Autodesk Inventor part; units mm, degrees
ref_plane "YZ Plane" through (0, 0, 0) normal (1, 0, 0) x (0, 1, 0)
ref_plane "XZ Plane" through (0, 0, 0) normal (0, 1, 0) x (-1, 0, 0)
ref_plane "XY Plane" through (0, 0, 0) normal (0, 0, 1) x (1, 0, 0)
sketch "スケッチ1" plane through (0, 0, 0) normal (0, 0, 1) x (1, 0, 0)
  circle A0 centre (0, 0) radius 2.75
  dimension "d0" = 5.5
extrude "押し出し1" add sketch "スケッチ1" along normal blind 3.6
sketch "スケッチ2" plane through (0, 0, 3.6) normal (0, 0, 1) x (1, 0, 0)
  circle A0 centre (0, 0) radius 1.5
  dimension "d3" = 3
extrude "押し出し2" add sketch "スケッチ2" along normal blind 15
thread "ねじ1"
sketch "スケッチ3" plane through (0, 0, 0) normal (0, 0, -1) x (-1, 0, 0)
  line L0 (0, -1.4434) -> (-1.25, -0.7217)
  line L1 (-1.25, -0.7217) -> (-1.25, 0.7217)
  line L2 (-1.25, 0.7217) -> (0, 1.4434)
  line L3 (0, 1.4434) -> (1.25, 0.7217)
  line L4 (1.25, 0.7217) -> (1.25, -0.7217)
  line L5 (1.25, -0.7217) -> (0, -1.4434)
  point P0 (0, 0)
  point P1 (0, 0)
  dimension "d8" = 2.5
extrude "押し出し3" cut sketch "スケッチ3" against normal blind 2
properties part number "Bolt_M3_15_for_SetCollar_d6" material "ステンレス鋼"
The model under review builds one solid part; all positions refer to its coordinate system, in mm. A direction names the side the tool comes from. Coordinates: 2 decimals unless noted, no trailing zeros. Write each loop counter-clockwise with the first axis right and the second up, starting at its lowest first coordinate (ties: lowest second). Pieces come first, ordered by that corner, then holes. Notation, with made-up numbers: (21.5, -17) - (65.5, -17) arc R19 cw to (65.5, 6) - close; hole circle Ø6 at (8.5, -38). An arc over 180 degrees is marked (long way). Answer in a Markdown table with one row per item. Add a question column.
Q1. Consider section B-B on x = 0.75. Give the boundary of the cut face in (y, z), then the cut area to 3 significant figures.
Q2. To check wall thickness, follow line 1 along Z through (x, y) = (-0.85, -1.55); line 2 along Z through (x, y) = (0.25, 0.45); line 3 along X through (y, z) = (0.4, 9.5). State the ranges of each line that lie inside material, in increasing order. Write a range as from..to.
Q3. Clearance check with a flat-ended pin moving along its axis: pin 1 (0.8 mm diameter, centred on x = 0, y = 0.5, fed in from -Z). State where the tip first meets the part, or that it passes through.
Q4. Consider section C-C on z = 8.75. Give the boundary of the cut face in (x, y), then the cut area to 3 significant figures.
Q5. For faces 1 (the face through (1.25, 0, 1)), 2 (the face through (0.6, 1.3, 0)), list the 3-axis set-ups (+Z, -Z, +X, -X, +Y, -Y) from which the entire face can be reached by the end or side of a thin tool; tool diameter is ignored.
Q6. Draft analysis for pull direction X (two halves, no side actions). For faces 3 (the face through (0.616, -1.088, 0.986)), 4 (the face through (-1.5, -0.07, 11)), 5 (the face through (1.2, -1.2, 3.6)), state which applies: +X half, -X half, draft (parallel to the pull), parting line (faces both ways), or undercut.
Q7. Consider section A-A on y = 0. Give the boundary of the cut face in (x, z), then the cut area to 3 significant figures.
Q8. Consider section D-D on x = -1.8. Give the boundary of the cut face in (y, z), then the cut area to 3 significant figures.
Answers below:
| question | item | result |
|---|---|---|
| 1 | outline | (-2.65, 0) - (-1.01, 0) - (-1.01, 2) - (1.01, 2) - (1.01, 0) - (2.65, 0) - (2.65, 3.6) - (1.3, 3.6) - (1.3, 18.6) - (-1.3, 18.6) - (-1.3, 3.6) - (-2.65, 3.6) - close |
| 1 | area | 54.0 mm² |
| 2 | line 1 | 0..3.6 |
| 2 | line 2 | 2..18.6 |
| 2 | line 3 | -1.45..1.45 |
| 3 | pin 1 | z = 2 |
| 4 | outline | circle Ø3 at (0, 0) |
| 4 | area | 7.07 mm² |
| 5 | face 1 | -Z |
| 5 | face 2 | -Z, +X, -X, +Y, -Y |
| 6 | face 3 | undercut |
| 6 | face 4 | parting line |
| 6 | face 5 | draft |
| 7 | outline | (-2.75, 0) - (-1.25, 0) - (-1.25, 2) - (1.25, 2) - (1.25, 0) - (2.75, 0) - (2.75, 3.6) - (1.5, 3.6) - (1.5, 18.6) - (-1.5, 18.6) - (-1.5, 3.6) - (-2.75, 3.6) - close |
| 7 | area | 59.8 mm² |
| 8 | outline | (-2.08, 0) - (2.08, 0) - (2.08, 3.6) - (-2.08, 3.6) - close |
| 8 | area | 15.0 mm² |
